```python
from build123d import *

# Parameters (mm, degrees)
COMPLETE_SKETCH_R                   = 1.6
BODY_DEPTH                          = 5
SMOOTHING_FILLET_R                  = 10
CUT_EXTRUDE1_START                  = -5
SKETCH1_R                           = 0.9
CUT_EXTRUDE1_DEPTH                  = 5
CUT_EXTRUDE2_START                  = -5
SKETCH1_4_W                         = 35
SKETCH1_4_H                         = 26
CUT_EXTRUDE2_DEPTH                  = 3.5
BOSS_EXTRUDE1_DEPTH                 = 24
ELEPHANTSFOOT_COMPENSATION_TOP_SIZE = 0.5
CHAMFER1_SIZE                       = 0.4


with BuildPart() as part:
    # complete_sketch → body (new body)
    with BuildSketch(Plane(origin=(0, 0, 0), x_dir=(1, 0, 0), z_dir=(0, 1, 0))):
        with BuildLine():
            Line((0, -20.5), (24, -20.5))
            ThreePointArc((24, -20.5), (35.188838333, -12.850097276), (39.5, 0))
            ThreePointArc((39.5, 0), (38.998281767, 8.558621384), (37.5, 17))
            ThreePointArc((37.5, 17), (32.5, 22), (27.5, 17))
            ThreePointArc((27.5, 17), (12, 14.321592614), (-3.5, 17))
            ThreePointArc((-3.5, 17), (-8.5, 22), (-13.5, 17))
            ThreePointArc((-13.5, 17), (-14.998281767, 8.558621384), (-15.5, 0))
            ThreePointArc((-15.5, 0), (-11.188838333, -12.850097276), (0, -20.5))
        make_face()
        with Locations(Location((24, 0, 0), (0, 0, 270))):
            Circle(COMPLETE_SKETCH_R, mode=Mode.SUBTRACT)
        with Locations(Location((-8.5, 17, 0), (0, 0, 270))):
            Circle(COMPLETE_SKETCH_R, mode=Mode.SUBTRACT)
        with Locations(Location((32.5, 17, 0), (0, 0, 270))):
            Circle(COMPLETE_SKETCH_R, mode=Mode.SUBTRACT)
    extrude(amount=BODY_DEPTH)

    # smoothing_fillet
    smoothing_fillet_edges = [part.edges().sort_by_distance(p)[0] for p in [
        (-3.5, 2.5, -17),
        (27.5, 2.5, -17),
    ]]
    fillet(smoothing_fillet_edges, radius=SMOOTHING_FILLET_R)

    # Sketch1 → Cut-Extrude1 (cut)
    with BuildSketch(Plane(origin=(0, 5, 0), x_dir=(1, 0, 0), z_dir=(0, 1, 0)).offset(CUT_EXTRUDE1_START)):
        with BuildLine():
            Line((31, -11), (31, 11))
            Line((31, 11), (19.196491673, 11))
            ThreePointArc((19.196491673, 11), (17.26, 9.5), (15.323508327, 11))
            Line((15.323508327, 11), (5.936491673, 11))
            ThreePointArc((5.936491673, 11), (4, 9.5), (2.063508327, 11))
            Line((2.063508327, 11), (0, 11))
            Line((0, 11), (0, -11))
            Line((0, -11), (2.063508327, -11))
            ThreePointArc((2.063508327, -11), (4, -9.5), (5.936491673, -11))
            Line((5.936491673, -11), (15.323508327, -11))
            ThreePointArc((15.323508327, -11), (17.26, -9.5), (19.196491673, -11))
            Line((19.196491673, -11), (31, -11))
        make_face()
        with Locations(Location((4, 11.5, 0), (0, 0, 270))):
            Circle(SKETCH1_R)
        with Locations(Location((17.26, 11.5, 0), (0, 0, 270))):
            Circle(SKETCH1_R)
        with Locations(Location((17.26, -11.5, 0), (0, 0, 270))):
            Circle(SKETCH1_R)
        with Locations(Location((4, -11.5, 0), (0, 0, 270))):
            Circle(SKETCH1_R)
    extrude(amount=CUT_EXTRUDE1_DEPTH, mode=Mode.SUBTRACT)

    # Sketch1<4> → Cut-Extrude2 (cut)
    with BuildSketch(Plane(origin=(0, 5, 0), x_dir=(1, 0, 0), z_dir=(0, 1, 0)).offset(CUT_EXTRUDE2_START)):
        with Locations((15.5, 0)):
            Rectangle(SKETCH1_4_W, SKETCH1_4_H)
    extrude(amount=CUT_EXTRUDE2_DEPTH, mode=Mode.SUBTRACT)

    # Sketch2 → Boss-Extrude1 (add)
    with BuildSketch(Plane(origin=(0, 0, 0), x_dir=(0, 0, -1), z_dir=(1, 0, 0))):
        with BuildLine():
            Line((-20.5, 0), (-23.5, 0))
            ThreePointArc((-23.5, 0), (-24.914213562, 0.585786438), (-25.5, 2))
            Line((-25.5, 2), (-25.5, 5))
            Line((-25.5, 5), (-22.5, 5))
            Line((-22.5, 5), (-22.5, 3))
            Line((-22.5, 3), (-20.5, 3))
            Line((-20.5, 3), (-20.5, 0))
        make_face()
    extrude(amount=BOSS_EXTRUDE1_DEPTH)

    # elephantsfoot_compensation top
    elephantsfoot_compensation_top_edges = [part.edges().sort_by_distance(p)[0] for p in [
        (33.926618039, 5, -21.792156192),
        (25.643793964, 5, -16.988490587),
        (38.998281767, 5, -8.558621384),
        (12, 5, -14.321592614),
        (35.188838333, 5, 12.850097276),
        (-1.643793964, 5, -16.988490587),
        (12, 5, 20.5),
        (-9.926618039, 5, -21.792156192),
        (-11.188838333, 5, 12.850097276),
        (-14.998281767, 5, -8.558621384),
        (24, 5, 24),
        (0, 5, 24),
        (12, 5, 25.5),
        (12, 5, 22.5),
    ]]
    chamfer(elephantsfoot_compensation_top_edges, length=ELEPHANTSFOOT_COMPENSATION_TOP_SIZE)

    # Chamfer1
    chamfer1_edges = [part.edges().sort_by_distance(p)[0] for p in [
        (12, 3, 22.5),
    ]]
    chamfer(chamfer1_edges, length=CHAMFER1_SIZE)


solid = part.part
```
Here's how the part is built. I have some questions about the finished solid (model axes, mm). A direction names the side the tool comes from. Give positions to 0.01 mm unless a question says otherwise; leave off trailing zeros. Use CSV: the item, a comma, the result in double quotes. Start each with the question number.
Item 1: On a 3-axis mill with a long thin cutter (end or side, diameter ignored), from which of +Z, -Z, +X, -X, +Y, -Y can I reach the whole of each face in a straight line? I mean faces 4 (the flat face through (12, 4, 22.5)), 5 (the cylindrical face through (-9.84, 2.218, -21.817)), 6 (the flat face through (0, 4, 0)), 7 (the cylindrical face through (-14.984, 2.218, -8.678)), 8 (the flat face through (15, 2, 13)). Say none if no direction works.
Item 2: Thinking about a two-plate mould opening in Z: for faces 1 (the cylindrical face through (31.53, 2.46, -18.27)), 2 (the flat face through (12, 5, 24)), 3 (the cylindrical face through (-11.3, 2.2, 12.7)), which applies, pulls with the +Z half, pulls with the -Z half, needs draft (parallel to the pull), parting line crosses it, or undercut?
Item 3: If I drill on probe 1 along Z at (x, y) = (11, 2.25); probe 2 along X at (y, z) = (4.45, 0.5); probe 3 along X at (y, z) = (4.1, -11.5), over which ranges is the centre line in solid material (lowest first)? Write a range as [from, to].
Item 4: Suppose I cut it at A-A (x = 4). Give the number of separate pieces and of enclosed holes in the cut face, and give its area (3 significant figures).
Item 5: I'm going to push flat-ended pins straight in: P1, Ø3, axis at x = -8.5, z = -17, coming from the +Y side; P2, Ø1.8, axis at x = 14.5, y = 1, coming from the +Z side; P3, Ø1.5, axis at y = 1, z = -5.5, coming from the -X side; P4, Ø2, axis at x = 4, z = -11.5, coming from the -Y side. Where does each tip first touch, or does it pass through?
Answer block:
1,face 4,"+X, -X, +Y"
1,face 5,"-Z, +Y, -Y"
1,face 6,"+Y, -Y"
1,face 7,"-Z, -X, +Y, -Y"
1,face 8,"-Y"
2,face 1,"undercut"
2,face 2,"needs draft"
2,face 3,"pulls with the +Z half"
3,probe 1,"z = [-14.33, -13], [13, 25.5]"
3,probe 2,"x = [-15.49, 0], [31, 39.49]"
3,probe 3,"x = [-14.59, 3.1], [4.9, 16.36], [18.16, 38.59]"
4,separate pieces,"4"
4,enclosed holes,"0"
4,area,"72.4 mm^2"
5,P1,"passes through"
5,P2,"stops at z = 25.5"
5,P3,"stops at x = -15.35"
5,P4,"stops at y = 3.5"
